The listing builds one solid part. Answer for the finished solid, in the listing's coordinates (mm). A direction names the side the tool comes from. Round coordinates to 2 decimals unless told otherwise and drop trailing zeros. Write each loop counter-clockwise with the first axis right and the second up, starting at its lowest first coordinate (ties: lowest second). Pieces come first, ordered by that corner, then holes. Notation, with made-up numbers: (67.25, -6.5) - (89.25, -6.5) arc R15 cw to (89.25, 11.5) - close; hole circle Ø10 at (80.5, 29.25). An arc over 180 degrees is marked (long way). Use a Markdown table: item, result. Add a question column.
1) Find the intervals of material crossed by probe 1 along X at (y, z) = (-0.5, 41); probe 2 along X at (y, z) = (1, 44); probe 3 along Y at (x, z) = (2.5, 40), in increasing order. Write a range as from..to.
2) A cutting plane is placed at B-B (y = 0). Give the vertices of the cut face in (x, z), then the cut area to 3 significant figures.
3) Determine the mould class of faces 3 (the flat face through (12, 0, 50.8)), 4 (the flat face through (-9.562, 0, 26)), 5 (the conical face through (-15.18, -11.64, -12.33)) for opening direction X: +X half, -X half, draft (parallel to the pull), parting line (faces both ways), or undercut.
4) Each of these flat-tipped pins is pushed along its axis until it touches: P1, Ø15.5, axis at x = -3.5, z = 24, coming from the -Y side; P2, Ø1, axis at x = -13.5, z = 1, coming from the +Y side; P3, Ø15.5, axis at x = -2.5, z = 28.5, coming from the +Y side. Where does it stop, or does it pass through?
5) A tool of negligible diameter and unlimited length cuts with its end or side. For faces 1 (the flat face through (0, 0, 0)), 2 (the flat face through (0, 0, -12.7)), from which of +Z, -Z, +X, -X, +Y, -Y can it reach the whole face along a straight path? Write none if from no direction.
6) A cutting plane is placed at C-C (x = 0). Give the vertices of the cut face in (y, z), then the cut area to 3 significant figures.
7) A cutting plane is placed at A-A (z = 43.5). Give the vertices of the cut face in (x, y).
```python
from build123d import *

# Parameters (mm, degrees)
F0_R     = 26.378327
F1_DEPTH = 12.7
F2_R     = 3.81
F3_SIZE  = 7.62
F4_R     = 17.961474
F5_DEPTH = 50.8
F6_W     = 19.1245
F6_H     = 18.48925
F7_DEPTH = 50.8


with BuildPart() as f1:
    # F0 (on Top) → F1 (new body)
    with BuildSketch(Plane.XY):
        Circle(F0_R)
    extrude(amount=-F1_DEPTH)

    # F2
    f2_edges = [f1.edges().sort_by_distance(p)[0] for p in [
        (-26.378327, 0, 0),
    ]]
    fillet(f2_edges, radius=F2_R)

    # F3
    f3_edges = [f1.edges().sort_by_distance(p)[0] for p in [
        (-26.378327, 0, -12.7),
    ]]
    chamfer(f3_edges, length=F3_SIZE)

    # F4 (on face) → F5 (join)
    with BuildSketch(Plane.XY):
        Circle(F4_R)
    extrude(amount=F5_DEPTH)

    # F6 (on face) → F7 (cut)
    with BuildSketch(Plane.XY.offset(50.8)):
        Rectangle(F6_W, F6_H)
    extrude(amount=-F7_DEPTH, mode=Mode.SUBTRACT)


solid = f1.part
```
Entries:
| question | item | result |
|---|---|---|
| 1 | probe 1 | x = -17.95..-9.56, 9.56..17.95 |
| 1 | probe 2 | x = -17.93..-9.56, 9.56..17.93 |
| 1 | probe 3 | y = -17.79..-9.24, 9.24..17.79 |
| 2 | outline | (-26.38, -5.08) - (-18.76, -12.7) - (18.76, -12.7) - (26.38, -5.08) - (26.38, -3.81) arc R3.81 ccw to (22.57, 0) - (17.96, 0) - (17.96, 50.8) - (9.56, 50.8) - (9.56, 0) - (-9.56, 0) - (-9.56, 50.8) - (-17.96, 50.8) - (-17.96, 0) - (-22.57, 0) arc R3.81 ccw to (-26.38, -3.81) - close |
| 2 | area | 1,460 mm² |
| 3 | face 3 | draft |
| 3 | face 4 | undercut |
| 3 | face 5 | parting line |
| 4 | P1 | stops at y = -17.96 |
| 4 | P2 | stops at y = 12.39 |
| 4 | P3 | stops at y = 17.96 |
| 5 | face 1 | +Z |
| 5 | face 2 | -Z, +X, -X, +Y, -Y |
| 6 | outline | (-26.38, -5.08) - (-18.76, -12.7) - (18.76, -12.7) - (26.38, -5.08) - (26.38, -3.81) arc R3.81 ccw to (22.57, 0) - (17.96, 0) - (17.96, 50.8) - (9.24, 50.8) - (9.24, 0) - (-9.24, 0) - (-9.24, 50.8) - (-17.96, 50.8) - (-17.96, 0) - (-22.57, 0) arc R3.81 ccw to (-26.38, -3.81) - close |
| 6 | area | 1,490 mm² |
| 7 | outline | circle Ø35.92 at (0, 0); hole (-9.56, -9.24) - (9.56, -9.24) - (9.56, 9.24) - (-9.56, 9.24) - close |
